Part model, mm, in its own coordinate system. Face numbers are marked on the shaded views. A direction names the side the tool comes from. Round coordinates to 2 decimals unless told otherwise and drop trailing zeros. Loops run counter-clockwise (first coordinate to the right, second up) from the corner with the lowest first, then second, coordinate; pieces in that order, holes last.
(1) Flat gauge pins, fed straight in: pin 1 (1.3 mm diameter, centred on x = 11.5, z = -1.5, fed in from +Y); pin 2 (4 mm diameter, centred on x = 15, y = -11, fed in from +Z); pin 3 (2.5 mm diameter, centred on x = -1.97, y = 16.89, fed in from -Z); pin 4 (11 mm diameter, centred on x = 4.5, y = 3.5, fed in from +Z). Where does each tip first touch, or does it go through?
(2) Tool access for the marked faces 1, 2 and 3: list every direction of +Z, -Z, +X, -X, +Y, -Y with a clear straight run to the whole face (end or side of a thin tool).
(3) Cut at A-A on y = 0. List the corners of the cut face in (x, z).
(4) Probe probe 1 along Y at (x, z) = (-8, -5.5); probe 2 along X at (y, z) = (0.5, -6.25); probe 3 along Y at (x, z) = (-6.5, -5.25). List the from-to ranges inside material, lowest first.
(5) Mould opens along X. For the marked faces 4, 5 and 6 say: +X half, -X half, draft (parallel to the pull), parting line (faces both ways), or undercut.
(6) Cut at D-D on y = 6. List the corners of the cut face in (x, z), then the cut area to 3 significant figures.
(7) Cut at C-C on z = -4.75. List the corners of the cut face in (x, y), then the cut area to 3 significant figures.
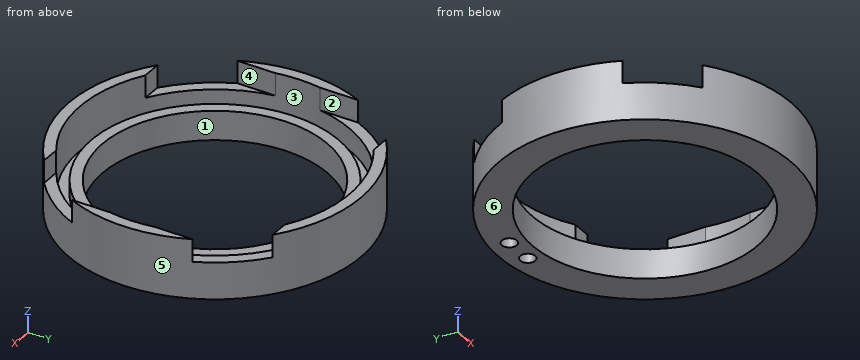
from build123d import *

# Parameters (mm, degrees)
F2_R     = 1
F3_DEPTH = 25
F4_W     = 35.5
F4_H     = 30.5
F5_DEPTH = 3


with BuildPart() as f1:
    # F0 (on Front) → F1 (revolve)
    with BuildSketch(Plane.XZ):
        Polygon((-15, -4), (-16.5, -4), (-16.5, -5.9), (-18, -5.9), (-18, 0), (-19.5, 0), (-19.5, -7.9), (-15, -7.9), align=None)
    revolve(axis=Axis((0, 0, -4.832979), (0, 0, -1)))

    # F2 (on face) → F3 (cut)
    with BuildSketch(Plane.XY.offset(-5.9)):
        with Locations((-1.971014, 16.885352)):
            Circle(F2_R)
        with Locations((1.971014, 16.885352)):
            Circle(F2_R)
    extrude(amount=-F3_DEPTH, mode=Mode.SUBTRACT)

    # F4 (on face) → F5 (cut)
    with BuildSketch(Plane.XY):
        Rectangle(F4_W, F4_H)
    extrude(amount=-F5_DEPTH, mode=Mode.SUBTRACT)


solid = f1.part
Final values:
1. pin 1: stops at y = 16.2
1. pin 2: stops at z = -3
1. pin 3: stops at z = -7.9
1. pin 4: passes through
2. face 1: +Z, -Z
2. face 2: +Z, +Y, -Y
2. face 3: +Z
3. outline: (-19.5, -7.9) - (-15, -7.9) - (-15, -4) - (-16.5, -4) - (-16.5, -5.9) - (-18, -5.9) - (-18, 0) - (-19.5, 0) - close; (15, -7.9) - (19.5, -7.9) - (19.5, 0) - (18, 0) - (18, -5.9) - (16.5, -5.9) - (16.5, -4) - (15, -4) - close
4. probe 1: y = -17.78 to -16.12, -14.43 to -12.69, 12.69 to 14.43, 16.12 to 17.78
4. probe 2: x = -19.49 to -14.99, 14.99 to 19.49
4. probe 3: y = -18.38 to -16.79, -15.17 to -13.52, 13.52 to 15.17, 16.79 to 18.38
5. face 4: undercut
5. face 5: parting line
5. face 6: draft
6. outline: (-18.55, -7.9) - (-13.75, -7.9) - (-13.75, -4) - (-15.37, -4) - (-15.37, -5.9) - (-16.97, -5.9) - (-16.97, -3) - (-17.75, -3) - (-17.75, 0) - (-18.55, 0) - close; (13.75, -7.9) - (18.55, -7.9) - (18.55, 0) - (17.75, 0) - (17.75, -3) - (16.97, -3) - (16.97, -5.9) - (15.37, -5.9) - (15.37, -4) - (13.75, -4) - close
6. area: 39.4 mm2
7. outline: circle Ø39 at (0, 0); circle Ø33 at (0, 0); hole circle Ø36 at (0, 0); hole circle Ø30 at (0, 0)
7. area: 325 mm2
